from build123d import *

# Parameters (mm, degrees)
SKETCH1_W           = 86
SKETCH1_H           = 23
BOSS_EXTRUDE1_DEPTH = 3.175
BOSS_EXTRUDE2_DEPTH = 3.175
SKETCH18_R          = 2.159
CUT_EXTRUDE2_DEPTH  = 127
SKETCH19_R          = 1.397
CUT_EXTRUDE3_DEPTH  = 47.652019249
SKETCH28_W          = 1.563549178
SKETCH28_H          = 8.443792612
BOSS_EXTRUDE4_DEPTH = 3.175
SKETCH27_W          = 57.315527743
SKETCH27_H          = 14.55620742
SKETCH27_W_2        = 22.489872753
CUT_EXTRUDE5_DEPTH  = 3.175
SKETCH29_W          = 13.689872798
SKETCH29_H          = 10.795
SKETCH29_W_2        = 13.689872764
CUT_EXTRUDE6_DEPTH  = 50.8
RIB3_REACH          = 68.958
SKETCH30_WALL_W     = 153.142504754
SKETCH30_WALL_H     = 2.54


with BuildPart() as part:
    # Sketch1 → Boss-Extrude1 (new body)
    with BuildSketch(Plane.XY):
        Rectangle(SKETCH1_W, SKETCH1_H)
    extrude(amount=-BOSS_EXTRUDE1_DEPTH)

    # Sketch3 → Boss-Extrude2 (add)
    with BuildSketch(Plane(origin=(0, -11.5, 0), x_dir=(-1, 0, 0), z_dir=(0, -1, 0))):
        Polygon((34.200000011, 0), (34.200000011, -10.795), (8.80000001, -10.795), (8.800000011, 0), align=None)
        Polygon((-34.200000011, 0), (-34.200000011, -10.795), (-8.80000001, -10.795), (-8.800000011, 0), align=None)
    extrude(amount=-BOSS_EXTRUDE2_DEPTH)

    # Sketch18 → Cut-Extrude2 (cut)
    with BuildSketch(Plane(origin=(0, 11.5, 0), x_dir=(1, 0, 0), z_dir=(0, 1, 0))):
        with Locations(Location((-14.626260209, -5.177433052, 0), (0, 0, 270))):
            Circle(SKETCH18_R)
        with Locations(Location((28.373739812, -5.177433052, 0), (0, 0, 90))):
            Circle(SKETCH18_R)
    extrude(amount=-CUT_EXTRUDE2_DEPTH, mode=Mode.SUBTRACT)

    # Sketch19 → Cut-Extrude3 (cut, through all)
    with BuildSketch(Plane(origin=(0, 0, -3.175), x_dir=(-1, 0, 0), z_dir=(0, 0, -1))):
        with Locations((-41.206, -8.579)):
            Circle(SKETCH19_R)
        with Locations((-18.9429, -6.801)):
            Circle(SKETCH19_R)
        with Locations((17.473, 8.7438)):
            Circle(SKETCH19_R)
        with Locations((39.952, -8.452)):
            Circle(SKETCH19_R)
    extrude(amount=-CUT_EXTRUDE3_DEPTH, mode=Mode.SUBTRACT)

    # Sketch28 → Boss-Extrude4 (add)
    with BuildSketch(Plane(origin=(0, 0, -3.175), x_dir=(-1, 0, 0), z_dir=(0, 0, -1))):
        with Locations((-43.781774589, -7.278103694)):
            Rectangle(SKETCH28_W, SKETCH28_H)
    extrude(amount=-BOSS_EXTRUDE4_DEPTH)

    # Sketch27 → Cut-Extrude5 (cut)
    with BuildSketch(Plane(origin=(0, 0, -3.175), x_dir=(-1, 0, 0), z_dir=(0, 0, -1))):
        with Locations((-14.342236128, 4.22189629)):
            Rectangle(SKETCH27_W, SKETCH27_H)
        with Locations((31.755063623, 4.22189629)):
            Rectangle(SKETCH27_W_2, SKETCH27_H)
    extrude(amount=-CUT_EXTRUDE5_DEPTH, mode=Mode.SUBTRACT)

    # Sketch29 → Cut-Extrude6 (cut)
    with BuildSketch(Plane(origin=(0, 11.5, 0), x_dir=(1, 0, 0), z_dir=(0, 1, 0))):
        with Locations((15.644936409, -5.3975)):
            Rectangle(SKETCH29_W, SKETCH29_H)
        with Locations((-27.355063629, -5.3975)):
            Rectangle(SKETCH29_W_2, SKETCH29_H)
    extrude(amount=-CUT_EXTRUDE6_DEPTH, mode=Mode.SUBTRACT)

    # Sketch30 wall → Rib3 (add, up to next)
    with BuildSketch(Plane(origin=(-20.510127247, -1.612609393, 5.3975), x_dir=(0, -0.779303981028, 0.626646076468), z_dir=(0, 0.626646076468, 0.779303981028)), mode=Mode.PRIVATE) as rib3_sk1:
        with Locations((0, 1.27)):
            Rectangle(SKETCH30_WALL_W, SKETCH30_WALL_H)
    rib3_tool1 = extrude(rib3_sk1.sketch, amount=-RIB3_REACH, mode=Mode.PRIVATE) - part.part
    add(rib3_tool1.solids().sort_by_distance((-20.510127247, -1.612609393, 5.3975))[0])


solid = part.part
Verification items for the finished model (mm, model axes). A direction names the side the tool comes from. Give positions to 0.01 mm unless a question says otherwise; leave off trailing zeros. Order: outer loops, then holes, each group sorted by start corner. A loop starts at its lowest first (then second) coordinate and runs counter-clockwise, first axis right, second up. Notation, with made-up numbers: M 19.25,-10.5 L 43.25,-10.5 A10 ccw 43.25,6.5 Z; hole C 12,86 d7. An arc over 180 degrees is marked long. Answer as a JSON object with one key per item and string values. Group by question number.
1) Mould release check, pull along Y, two halves, no side actions. Record for faces 5 (the face through (-19.222, -1.519, 5.322)), 6 (the face through (26.233, -9.89, 5.458)), 7 (the face through (42.2, -7.6, -1.6)): released by +Y, released by -Y, zero draft, split by the parting line, or undercut.
2) Cross-section at D-D (x = -8). Enter the section's corners in (y, z) (3 decimals), then the cut area to 3 significant figures.
3) Cross-section at B-B (z = -2). Enter the section's corners in (x, y).
4) Cross-section at C-C (y = 0.5). Enter the section's corners in (x, z) (3 decimals).
5) Cross-section at A-A (z = 4.5). Enter the section's corners in (x, y) (3 decimals), then the cut area to 3 significant figures.
6) Depth check by flat-ended pin: pin 1 Ø3.5 at (x, z) = (17.5, -2) entering from +Y; pin 2 Ø3 at (y, z) = (3.5, -1.5) entering from -X; pin 3 Ø10 at (x, y) = (3, -0.5) entering from +Z; pin 4 Ø3 at (x, y) = (28, -2.5) entering from -Z (3 decimals). Enter the tip coordinate at first touch or a pass-through.
7) Scan lines: line 1 along X through (y, z) = (-5.75, 1); line 2 along X through (y, z) = (1.5, -0.5); line 3 along Y through (x, z) = (26, 7.75) (3 decimals). Record each from-to range of solid material in increasing order. Write a range as [from, to].
8) Access from +Z, -Z, +X, -X, +Y, -Y to the whole of each face (thin tool, end or side, straight path). Record for faces 1 (the face through (22.49, -10, 5)), 2 (the face through (34.2, -10, 5)), 3 (the face through (-17.97, -4, 3)), 4 (the face through (16, -3.056, -2)).
Result sheet:
{
 "1": {"face 5": "released by +Y", "face 6": "zero draft", "face 7": "undercut"},
 "2": {"outline": "M -11.5,-3.175 L -3.056,-3.175 L -3.056,0 L -11.5,0 Z", "area": "26.8 mm2"},
 "3": {"outline": "M -43,-11.5 L 44.56,-11.5 L 44.56,-3.06 L -14.32,-3.06 L -14.32,11.5 L -20.51,11.5 L -20.51,-3.06 L -43,-3.06 Z; hole C -39.95,-8.45 d2.79; hole C -17.47,8.74 d2.79; hole C 18.94,-6.8 d2.79; hole C 41.21,-8.58 d2.79"},
 "4": {"outline": "M -20.51,-3.175 L -14.316,-3.175 L -14.316,0 L -17.97,0 L -17.97,3.699 L -20.51,3.699 Z"},
 "5": {"outline": "M -20.51,-11.5 L -16.676,-11.5 L -16.676,-8.325 L -17.97,-8.325 L -17.97,-0.496 L -20.51,-0.496 Z; M -12.576,-11.5 L -8.8,-11.5 L -8.8,-8.325 L -12.576,-8.325 Z; M 22.49,-11.5 L 26.324,-11.5 L 26.324,-8.325 L 22.49,-8.325 Z; M 30.424,-11.5 L 34.2,-11.5 L 34.2,-8.325 L 30.424,-8.325 Z", "area": "68.2 mm2"},
 "6": {"pin 1": "stops at y = -3.06", "pin 2": "stops at x = -20.51", "pin 3": "stops at z = 0", "pin 4": "stops at z = -3.175"},
 "7": {"line 1": "x = [-20.51, -17.97]", "line 2": "x = [-20.51, -14.32]", "line 3": "y = [-11.5, -8.325]"},
 "8": {"face 1": "+Z, +Y, -Y", "face 2": "+Z, +X, +Y, -Y", "face 3": "+Z, +X, +Y", "face 4": "+Z, -Z, +X, +Y"}
}
